```python
from build123d import *

# Parameters (mm, degrees)
SKETCH1_R           = 2.000000064
BOSS_EXTRUDE1_DEPTH = 177.8
SKETCH3_R           = 6.35
SKETCH3_R_2         = 2.000000064
BOSS_EXTRUDE3_DEPTH = 7.9375
SKETCH5_W           = 0.889
SKETCH5_H           = 1.0033


with BuildPart() as part:
    # Sketch1 → Boss-Extrude1 (new, symmetric)
    with BuildSketch(Plane.XY):
        with BuildLine():
            ThreePointArc((0.93173274, 6.79441227), (0, 6.858), (-0.93173274, 6.79441227))
            Line((-0.93173274, 6.79441227), (-5.41826726, 4.204110358))
            ThreePointArc((-5.41826726, 4.204110358), (-5.939202219, 3.429), (-6.35, 2.590301913))
            Line((-6.35, 2.590301913), (-6.35, -2.590301913))
            ThreePointArc((-6.35, -2.590301913), (-5.939202219, -3.429), (-5.41826726, -4.204110358))
            Line((-5.41826726, -4.204110358), (-0.93173274, -6.79441227))
            ThreePointArc((-0.93173274, -6.79441227), (0, -6.858), (0.93173274, -6.79441227))
            Line((0.93173274, -6.79441227), (5.41826726, -4.204110358))
            ThreePointArc((5.41826726, -4.204110358), (5.939202219, -3.429), (6.35, -2.590301913))
            Line((6.35, -2.590301913), (6.35, 2.590301913))
            ThreePointArc((6.35, 2.590301913), (5.939202219, 3.429), (5.41826726, 4.204110358))
            Line((5.41826726, 4.204110358), (0.93173274, 6.79441227))
        make_face()
        Circle(SKETCH1_R, mode=Mode.SUBTRACT)
    extrude(amount=BOSS_EXTRUDE1_DEPTH, both=True)

    # Sketch3 → Boss-Extrude3 (add)
    with BuildSketch(Plane.XY.offset(177.8)):
        Circle(SKETCH3_R)
        Circle(SKETCH3_R_2, mode=Mode.SUBTRACT)
    boss_extrude3 = extrude(amount=BOSS_EXTRUDE3_DEPTH)

    # Mirror1: Boss-Extrude3 across plane
    add(boss_extrude3.mirror(Plane.XY))

    # Sketch5 → Cut-Revolve1 (revolve, cut)
    with BuildSketch(Plane(origin=(0, 0, 0), x_dir=(0, 0, -1), z_dir=(1, 0, 0)), mode=Mode.PRIVATE) as cut_revolve1_sk:
        with Locations((-117.9195, 6.35635)):
            Rectangle(SKETCH5_W, SKETCH5_H)
    revolve(cut_revolve1_sk.sketch.rotate(Axis((0, 0, 0), (0, 0, -1)), 90), axis=Axis((0, 0, 0), (0, 0, -1)), mode=Mode.SUBTRACT)


solid = part.part
```
CAD build for the part. Positions are in the model's coordinates, mm. A direction names the side the tool comes from. Coordinates: 2 decimals unless noted, no trailing zeros. Order: outer loops, then holes, each group sorted by start corner. A loop starts at its lowest first (then second) coordinate and runs counter-clockwise, first axis right, second up. Notation, with made-up numbers: (-2.5, 3) - (7.5, 3) arc R6 cw to (7.5, 9) - close; hole circle Ø7 at (41.25, -20). An arc over 180 degrees is marked (long way). Answer in a Markdown table with one row per item.
1. Pull direction Z, two halves, no side cores. Call faces 1 (the face through (-5.85, -0.26, 117.91)), 2 (the face through (-2, 2, -185.738)), 3 (the face through (-1.38, -6.2, 181.71)): +Z half, -Z half, draft (parallel to the pull), parting line (faces both ways), or undercut.
Answer:
| item | result |
|---|---|
| face 1 | undercut |
| face 2 | -Z half |
| face 3 | draft |
2. Flat gauge pins, fed straight in: P1, Ø2, axis at y = -5, z = 108.5, coming from the +X side; P2, Ø1, axis at x = -5.5, y = -3.5, coming from the +Z side; P3, Ø1, axis at x = 3, z = -121.5, coming from the -Y side. Where does each tip first touch, or does it go through?
Answer:
| item | result |
|---|---|
| P1 | x = 5.57 |
| P2 | z = 185.74 |
| P3 | y = -5.89 |
3. Slice it at A-A, the plane z = 126.5. List the corners of the cut face in (x, y).
Answer:
| item | result |
|---|---|
| outline | (-6.35, -2.59) arc R6.86 ccw to (-5.42, -4.2) - (-0.93, -6.79) arc R6.86 ccw to (0.93, -6.79) - (5.42, -4.2) arc R6.86 ccw to (6.35, -2.59) - (6.35, 2.59) arc R6.86 ccw to (5.42, 4.2) - (0.93, 6.79) arc R6.86 ccw to (-0.93, 6.79) - (-5.42, 4.2) arc R6.86 ccw to (-6.35, 2.59) - close; hole circle Ø4 at (0, 0) |
4. 3-axis set-ups, long thin cutter, end or side, ignore diameter. For faces 4 (the face through (6, -2, 117.475)), 5 (the face through (-1.38, -6.2, -181.71)), 6 (the face through (-2, 2, 185.738)): which of +Z, -Z, +X, -X, +Y, -Y reach the whole face in a straight line?
Answer:
| item | result |
|---|---|
| face 4 | none |
| face 5 | -Z |
| face 6 | +Z, +X, -X, +Y, -Y |
5. Drill centre lines: L1, parallel to Y at x = -1.75, z = -140; L2, parallel to Y at x = -0.25, z = -115; L3, parallel to Z at x = -3.5, y = 4.75 (1 decimal). Where is each one in solid material? Low to high. Write a range as from..to.
Answer:
| item | result |
|---|---|
| L1 | -6.32..-0.97, 0.97..6.32 |
| L2 | -6.85..-1.98, 1.98..6.85 |
| L3 | -185.7..117.5, 118.4..185.7 |
